Part model, mm, in its own coordinate system. Face numbers are marked on the shaded views. A direction names the side the tool comes from. Coordinates: 2 decimals unless noted, no trailing zeros. Write each loop counter-clockwise with the first axis right and the second up, starting at its lowest first coordinate (ties: lowest second). Pieces come first, ordered by that corner, then holes. Notation, with made-up numbers: (-18.75, -2) -> (36.25, -2) arc R31 ccw to (36.25, 28) -> close; hole circle Ø9 at (-1, 41.5). An arc over 180 degrees is marked (long way). One line per question, with ' | ' between items. Start each with the question number.
Item 1: 3-axis set-ups, long thin cutter, end or side, ignore diameter. For the marked faces 5, 6 and 7: which of +Z, -Z, +X, -X, +Y, -Y reach the whole face in a straight line?
Item 2: Saw through at D-D (z = -32.5). List the corners of the cut face in (x, y).
Item 3: Two-plate mould, pull along X, no slides. Class the marked faces 1, 2, 3 and 4: pulls with the +X half, pulls with the -X half, needs draft (parallel to the pull), parting line crosses it, or undercut.
Item 4: Saw through at B-B (y = 36). List the corners of the cut face in (x, z), and give its area (3 significant figures).
Item 5: Saw through at A-A (x = -21). List the corners of the cut face in (y, z).
Item 6: Saw through at C-C (x = 14). List the corners of the cut face in (y, z).
Item 7: Pin check, flat tips, straight feed: pin 1 (4.5 mm diameter, centred on x = 9, y = 30, fed in from +Z); pin 2 (4.5 mm diameter, centred on y = 27, z = 13.5, fed in from +X). Stop position of each tip, or through.
Item 8: Probe probe 1 along Y at (x, z) = (-7, -3); probe 2 along Z at (x, y) = (17.5, 29); probe 3 along Y at (x, z) = (-17, 32). List the from-to ranges inside material, lowest first. Write a range as [from, to].
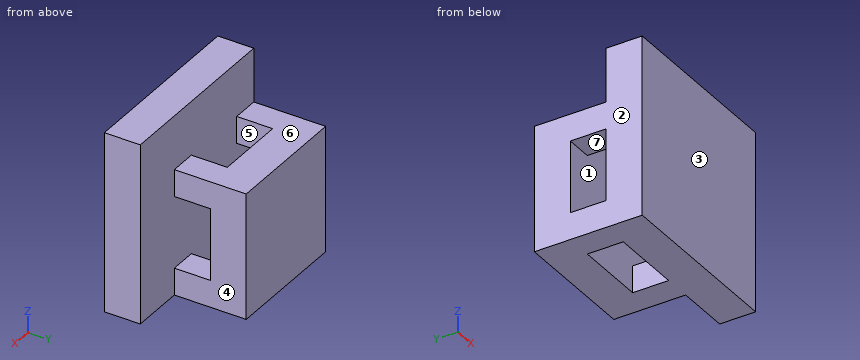
from build123d import *

# Parameters (mm, degrees)
CROQUIS1_W              = 100
CROQUIS1_H              = 100
SALIENTE_EXTRUIR1_DEPTH = 20
CROQUIS2_W              = 15
CROQUIS2_H              = 15
SALIENTE_EXTRUIR2_DEPTH = 20
CROQUIS3_W              = 70
CROQUIS3_H              = 70
SALIENTE_EXTRUIR3_DEPTH = 20


with BuildPart() as part:
    # Croquis1 → Saliente-Extruir1 (new body)
    with BuildSketch(Plane(origin=(0, 0, 0), x_dir=(1, 0, 0), z_dir=(0, 1, 0))):
        Rectangle(CROQUIS1_W, CROQUIS1_H)
    extrude(amount=SALIENTE_EXTRUIR1_DEPTH)

    # Croquis2 → Saliente-Extruir2 (add)
    with BuildSketch(Plane(origin=(0, 20, 0), x_dir=(1, 0, 0), z_dir=(0, 1, 0))):
        with Locations((-42.5, -12.5)):
            Rectangle(CROQUIS2_W, CROQUIS2_H)
        with Locations((-42.5, 42.5)):
            Rectangle(CROQUIS2_W, CROQUIS2_H)
        with Locations((12.5, 42.5)):
            Rectangle(CROQUIS2_W, CROQUIS2_H)
        with Locations((12.5, -12.5)):
            Rectangle(CROQUIS2_W, CROQUIS2_H)
    extrude(amount=SALIENTE_EXTRUIR2_DEPTH)

    # Croquis3 → Saliente-Extruir3 (add)
    with BuildSketch(Plane(origin=(0, 40, 0), x_dir=(1, 0, 0), z_dir=(0, 1, 0))):
        with Locations((-15, 15)):
            Rectangle(CROQUIS3_W, CROQUIS3_H)
    extrude(amount=SALIENTE_EXTRUIR3_DEPTH)


solid = part.part
From the geometry:
1) face 5: +Z, -Z | face 6: +Z, +X, -X, +Y | face 7: +X, -X
2) outline: (-50, 0) -> (50, 0) -> (50, 20) -> (-50, 20) -> close; (-50, 40) -> (20, 40) -> (20, 60) -> (-50, 60) -> close
3) face 1: undercut | face 2: pulls with the -X half | face 3: needs draft | face 4: pulls with the +X half
4) outline: (-50, -50) -> (-35, -50) -> (-35, -35) -> (-50, -35) -> close; (-50, 5) -> (-35, 5) -> (-35, 20) -> (-50, 20) -> close; (5, -50) -> (20, -50) -> (20, -35) -> (5, -35) -> close; (5, 5) -> (20, 5) -> (20, 20) -> (5, 20) -> close | area: 900 mm2
5) outline: (0, -50) -> (20, -50) -> (20, 50) -> (0, 50) -> close; (40, -50) -> (60, -50) -> (60, 20) -> (40, 20) -> close
6) outline: (0, -50) -> (60, -50) -> (60, 20) -> (20, 20) -> (20, 50) -> (0, 50) -> close; hole (20, -35) -> (40, -35) -> (40, 5) -> (20, 5) -> close
7) pin 1: z = 20 | pin 2: x = 20
8) probe 1: [0, 20], [40, 60] | probe 2: [-50, -35], [5, 20] | probe 3: [0, 20]
